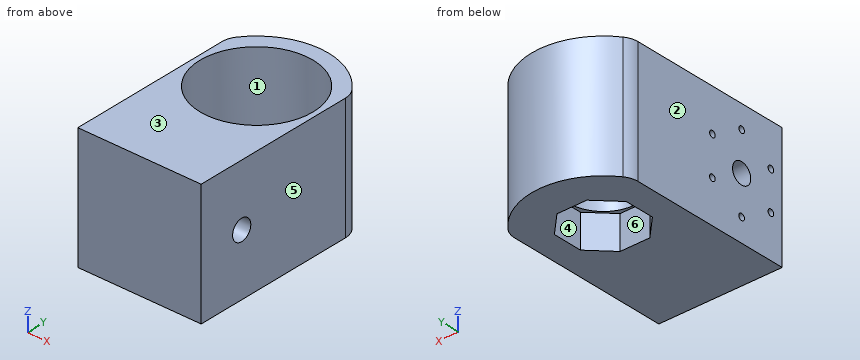
```python
from build123d import *

# Parameters (mm, degrees)
SKETCH1_W           = 76.2
SKETCH1_H           = 76.2
BOSS_EXTRUDE1_DEPTH = 127
SKETCH3_R           = 34.925
CUT_EXTRUDE1_DEPTH  = 47.625
CUT_EXTRUDE3_DEPTH  = 20.6375
CUT_EXTRUDE4_REACH  = 145.763
SKETCH6_R           = 20.955
CUT_EXTRUDE5_START  = -76.2
CUT_EXTRUDE5_DEPTH  = 76.2
FILLET1_R           = 12.7
SKETCH8_R           = 6.4135
CUT_EXTRUDE6_DEPTH  = 153.928251151
CIRPATTERN1_COUNT   = 6


with BuildPart() as part:
    # Sketch1 → Boss-Extrude1 (new body)
    with BuildSketch(Plane(origin=(0, 0, 0), x_dir=(1, 0, 0), z_dir=(0, 1, 0))):
        Rectangle(SKETCH1_W, SKETCH1_H)
    extrude(amount=BOSS_EXTRUDE1_DEPTH)

    # Sketch3 → Cut-Extrude1 (cut)
    with BuildSketch(Plane.XY.offset(38.1)):
        with Locations((0, 82.55)):
            Circle(SKETCH3_R)
    extrude(amount=-CUT_EXTRUDE1_DEPTH, mode=Mode.SUBTRACT)

    # Sketch5 → Cut-Extrude3 (cut)
    with BuildSketch(Plane(origin=(0, 0, -38.1), x_dir=(-1, 0, 0), z_dir=(0, 0, -1))):
        Polygon((22.225, 73.344103576), (22.225, 91.755896424), (9.205896424, 104.775), (-9.205896424, 104.775), (-22.225, 91.755896424), (-22.225, 73.344103576), (-9.205896424, 60.325), (9.205896424, 60.325), align=None)
    extrude(amount=-CUT_EXTRUDE3_DEPTH, mode=Mode.SUBTRACT)

    # Sketch6 → Cut-Extrude4 (cut, up to next)
    with BuildSketch(Plane(origin=(0, 0, -17.4625), x_dir=(-1, 0, 0), z_dir=(0, 0, -1)), mode=Mode.PRIVATE) as cut_extrude4_sk1:
        with Locations((0, 82.55)):
            Circle(SKETCH6_R)
    cut_extrude4_tool1 = extrude(cut_extrude4_sk1.sketch, amount=-CUT_EXTRUDE4_REACH, mode=Mode.PRIVATE) & part.part
    add(cut_extrude4_tool1.solids().sort_by_distance((0, 82.55, -17.4625))[0], mode=Mode.SUBTRACT)

    # Sketch7 → Cut-Extrude5 (cut)
    with BuildSketch(Plane.XY.offset(38.1).offset(CUT_EXTRUDE5_START)):
        with BuildLine():
            Line((-38.1, 105.445250599), (-38.1, 130.845250599))
            Line((-38.1, 130.845250599), (38.1, 130.845250599))
            Line((38.1, 130.845250599), (38.1, 105.445250599))
            ThreePointArc((38.1, 105.445250599), (0, 127), (-38.1, 105.445250599))
        make_face()
    extrude(amount=CUT_EXTRUDE5_DEPTH, mode=Mode.SUBTRACT)

    # Fillet1
    fillet1_edges = [part.edges().sort_by_distance(p)[0] for p in [
        (-38.1, 105.445250599, 0),
        (38.1, 105.445250599, 0),
    ]]
    fillet(fillet1_edges, radius=FILLET1_R)

    # Sketch8 → Cut-Extrude6 (cut, through all)
    with BuildSketch(Plane(origin=(38.1, 0, 0), x_dir=(0, 0, -1), z_dir=(1, 0, 0))):
        with Locations((0, 28.575)):
            Circle(SKETCH8_R)
    extrude(amount=-CUT_EXTRUDE6_DEPTH, mode=Mode.SUBTRACT)

    # Sketch12 → #10 (0.1935) Diameter Hole1 (revolve, cut)
    with BuildSketch(Plane(origin=(-38.1, 28.575, 23.8125), x_dir=(0, 0, 1), z_dir=(0, 1, 0))):
        Polygon((0, 0), (0, 10.717332791), (1.984375, 9.525), (1.984375, 0), align=None)
    f_10_0_1935_diameter_hole1 = revolve(axis=Axis((-44.45, 28.575, 23.8125), (1, 0, 0)), mode=Mode.SUBTRACT)

    # CirPattern1: #10 (0.1935) Diameter Hole1 ×6 about axis
    cirpattern1_axis = Axis((0, 28.575, 0), (1, 0, 0))
    for i in range(1, CIRPATTERN1_COUNT):
        add(f_10_0_1935_diameter_hole1.rotate(cirpattern1_axis, i * 360 / CIRPATTERN1_COUNT), mode=Mode.SUBTRACT)


solid = part.part
```
For this review, take the finished solid that the model builds, in its own axes (mm). Face numbers are marked on the shaded views. A direction names the side the tool comes from. Coordinates: 2 decimals unless noted, no trailing zeros. Write each loop counter-clockwise with the first axis right and the second up, starting at its lowest first coordinate (ties: lowest second). Pieces come first, ordered by that corner, then holes. Notation, with made-up numbers: (-25, 85) - (-9, 85) arc R23 cw to (-9, 96) - close; hole circle Ø9 at (79, -32). An arc over 180 degrees is marked (long way). Put each result on its own line as item: value.
1. Add section D-D, the plane x = -19.5. Give the boundary of the cut face in (y, z) (1 decimal), then the cut area to 3 significant figures.
Values found:
outline: (0, -38.1) - (70.6, -38.1) - (70.6, -17.5) - (74.9, -17.5) - (74.9, -9.5) - (53.6, -9.5) - (53.6, 38.1) - (0, 38.1) - close; (90.2, -17.5) - (94.5, -17.5) - (94.5, -38.1) - (122.5, -38.1) - (122.5, 38.1) - (111.5, 38.1) - (111.5, -9.5) - (90.2, -9.5) - close; hole circle Ø12.8 at (28.6, 0)
area: 5,830 mm²
2. Mouldability with a two-part tool opening along X and no side actions: class the marked faces 1, 2, 3 and 4 as released by +X, released by -X, zero draft, split by the parting line, or undercut.
Values found:
face 1: undercut
face 2: released by -X
face 3: zero draft
face 4: undercut
3. Machinability: for the marked faces 5 and 6, which of the approach directions +Z, -Z, +X, -X, +Y, -Y give a long, thin tool a straight path to every point of the face, cutting with its end or side? Answer none if there is none.
Values found:
face 5: +Z, -Z, +X, +Y, -Y
face 6: -Z
4. Add section B-B, the plane y = 82.55. Give the boundary of the cut face in (x, z) (1 decimal).
Values found:
outline: (-38.1, -38.1) - (-22.2, -38.1) - (-22.2, -17.5) - (-21, -17.5) - (-21, -9.5) - (-34.9, -9.5) - (-34.9, 38.1) - (-38.1, 38.1) - close; (21, -17.5) - (22.2, -17.5) - (22.2, -38.1) - (38.1, -38.1) - (38.1, 38.1) - (34.9, 38.1) - (34.9, -9.5) - (21, -9.5) - close
5. Add section A-A, the plane z = 0. Count the separate pieces of the cut face and the enclosed holes in it, then the cut area to 3 significant figures.
Values found:
separate pieces: 2
enclosed holes: 1
area: 4,380 mm²
6. For pin 1 (12 mm diameter, centred on x = 30, z = 15, fed in from +Y); pin 2 (2.5 mm diameter, centred on y = 28.57, z = -23.81, fed in from -X); pin 3 (12 mm diameter, centred on x = -6.5, y = 67, fed in from +Z) (3 decimals), all flat-tipped, find the tip position at first contact; note any pin that passes through.
Values found:
pin 1: y = 119.96
pin 2: x = -28.14
pin 3: z = -9.525
7. Add section C-C, the plane z = -27.5. Give the boundary of the cut face in (x, y) (3 decimals).
Values found:
outline: (-38.1, 0) - (38.1, 0) - (38.1, 101.6) arc R12.7 ccw to (35.56, 109.22) arc R44.45 ccw to (-35.56, 109.22) arc R12.7 ccw to (-38.1, 101.6) - close; hole (-22.225, 73.344) - (-9.206, 60.325) - (9.206, 60.325) - (22.225, 73.344) - (22.225, 91.756) - (9.206, 104.775) - (-9.206, 104.775) - (-22.225, 91.756) - close
8. Wall thickness on probe 1 along X at (y, z) = (90.5, -32) (3 decimals); probe 2 along X at (y, z) = (82, 12); probe 3 along Y at (x, z) = (29, 2): over which ranges is each line inside the solid? List them lowest first.
Values found:
probe 1: -38.1 to -22.225, 22.225 to 38.1
probe 2: -38.1 to -34.92, 34.92 to 38.1
probe 3: 0 to 22.48, 34.67 to 63.09, 102.01 to 116.24
